Part model, mm, in its own coordinate system. Face numbers are marked on the shaded views. Coordinates: 2 decimals unless noted, no trailing zeros. Order: outer loops, then holes, each group sorted by start corner. A loop starts at its lowest first (then second) coordinate and runs counter-clockwise, first axis right, second up.
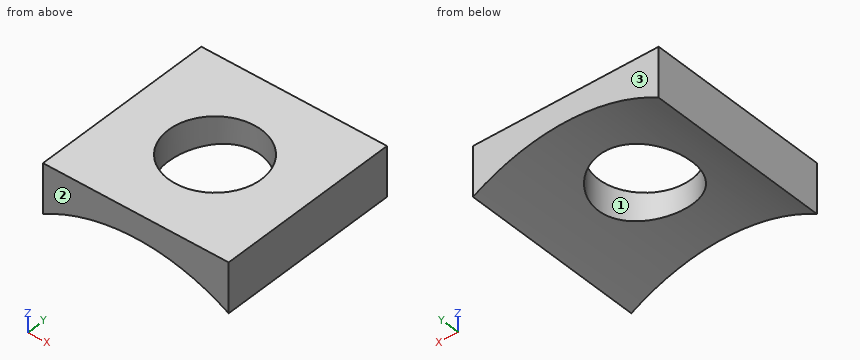
from build123d import *

# Parameters (mm, degrees)
F1_DEPTH = 100
F3_D     = 50


with BuildPart() as f1:
    # F0 (on Front) → F1 (new body)
    with BuildSketch(Plane.XZ):
        with BuildLine():
            ThreePointArc((-50, -13.39746), (0, 0), (50, -13.39746))
            Line((50, -13.39746), (50, 13.39746))
            Line((50, 13.39746), (-50, 13.39746))
            Line((-50, 13.39746), (-50, -13.39746))
        make_face()
    extrude(amount=F1_DEPTH)

    # F3 (through all)
    with Locations(Plane.XY.offset(13.39746)):
        with Locations((0, -50)):
            Hole(F3_D / 2)


solid = f1.part
Q1. Wall check: line 1 along X through (y, z) = (-50, 4.5); line 2 along Y through (x, z) = (0, 0.75); line 3 along X through (y, z) = (-69, 1.5). Give the ranges that are in metal, low to high.
Results list:
line 1: x = -50 to -25, 25 to 50
line 2: y = -100 to -75, -25 to 0
line 3: x = -50 to -16.25, 16.25 to 50
Q2. Cut at B-B on y = -50. Write the cut outline in (x, z), and give its area (3 significant figures).
Results list:
outline: (-50, -13.4) arc R100 cw to (-25, -3.18) - (-25, 13.4) - (-50, 13.4) - close; (25, -3.18) arc R100 cw to (50, -13.4) - (50, 13.4) - (25, 13.4) - close
area: 1,050 mm2
Q3. Cut at A-A on x = 0. Write the cut outline in (y, z).
Results list:
outline: (-100, 0) - (-75, 0) - (-75, 13.4) - (-100, 13.4) - close; (-25, 0) - (0, 0) - (0, 13.4) - (-25, 13.4) - close
Q4. Cut at C-C on z = 7. Write the cut outline in (x, y).
Results list:
outline: (-50, -100) - (50, -100) - (50, 0) - (-50, 0) - close; hole circle Ø50 at (0, -50)
Q5. Cut at D-D on y = -20. Write the cut outline in (x, z).
Results list:
outline: (-50, -13.4) arc R100 cw to (50, -13.4) - (50, 13.4) - (-50, 13.4) - close
Q6. Mould opens along Y. For the marked faces 1, 2 and 3 say: pulls with the +Y half, pulls with the -Y half, needs draft (parallel to the pull), parting line crosses it, or undercut.
Results list:
face 1: undercut
face 2: pulls with the -Y half
face 3: pulls with the +Y half
